from build123d import *

# Parameters (mm, degrees)
F0_W     = 152.4
F0_H     = 76.2
F1_DEPTH = 50.8
F3_DEPTH = 152.401
F5_DEPTH = 76.201
F6_W     = 76.2
F6_H     = 12.7
F7_DEPTH = 76.201


with BuildPart() as f1:
    # F0 (on Top) → F1 (new body)
    with BuildSketch(Plane.XY):
        Rectangle(F0_W, F0_H)
    extrude(amount=F1_DEPTH)

    # F2 (on face) → F3 (cut, through all)
    with BuildSketch(Plane.YZ.offset(76.2)):
        Polygon((25.40207, 12.7), (-25.4, 12.7), (-12.7, 0), (12.70207, 0), align=None)
    extrude(amount=-F3_DEPTH, mode=Mode.SUBTRACT)

    # F4 (on face) → F5 (cut, through all)
    with BuildSketch(Plane.XZ.offset(38.1)):
        Polygon((-25.4, 50.8), (-50.8, 50.8), (-50.8, 38.1), (-63.5, 38.1), (-63.5, 25.4), (-12.7, 25.4), (-12.7, 38.1), (-25.4, 38.1), align=None)
    extrude(amount=-F5_DEPTH, mode=Mode.SUBTRACT)

    # F6 (on face) → F7 (cut, through all)
    with BuildSketch(Plane.XZ.offset(38.1)):
        with Locations((38.1, 44.45)):
            Rectangle(F6_W, F6_H)
        Polygon((0, 38.1), (0, 50.8), (-7.272681, 50.8), align=None)
    extrude(amount=-F7_DEPTH, mode=Mode.SUBTRACT)


solid = f1.part
Can you work these out from the model? Positions are in its coordinate system, mm. A direction names the side the tool comes from. Give positions to 0.01 mm unless a question says otherwise; leave off trailing zeros. Order: outer loops, then holes, each group sorted by start corner. A loop starts at its lowest first (then second) coordinate and runs counter-clockwise, first axis right, second up. Notation, with made-up numbers: M 36.5,55 L 90.5,55 A13 ccw 90.5,73 Z; hole C -16,-5 d2. An arc over 180 degrees is marked long. Use one line per item in the form item = value. Start each with the question number.
Item 1: For faces 1 (the flat face through (-3.69, -0.53, 44.54)), 2 (the flat face through (-57, -1, 38.1)), 3 (the flat face through (-50.8, -1, 45)), 4 (the flat face through (1.1, 19, 6.3)), which set-ups out of +Z, -Z, +X, -X, +Y, -Y let a thin tool reach every point of the face, with its end or its side?
Item 2: If I drill on line 1 along X through (y, z) = (-8, 32.5); line 2 along Z through (x, y) = (-59.5, -4); line 3 along Z through (x, y) = (-18, 24.5), over which ranges is the centre line in solid material (lowest first)?
Item 3: If we section it at A-A (x = -52.5): Write out the boundary of the cut face in (y, z), then the cut area to 3 significant figures.
Item 4: If we section it at B-B (z = 8): Write out the boundary of the cut face in (x, y).
Item 5: If we section it at D-D (x = -10): Write out the boundary of the cut face in (y, z).
Item 6: If we section it at C-C (y = 18.5): Write out the boundary of the cut face in (x, z), then the cut area to 3 significant figures.
Item 7: We'd pull the mould along Y, two halves only. Please class faces 5 (the flat face through (-1, -38.1, 19)), 6 (the flat face through (1, 0, 12.7)), 7 (the flat face through (-1, -25, 0)): +Y half, -Y half, draft (parallel to the pull), parting line (faces both ways), or undercut.
Item 8: Will these pins go through, and if not, where does the flat tip stop? pin 1 Ø4 at (x, y) = (-20.5, -2) entering from -Z; pin 2 Ø3 at (x, y) = (-29, 11.5) entering from +Z; pin 3 Ø2 at (x, y) = (5, 26.5) entering from +Z.
Outcome:
q1.face_1 = +Z, +X, +Y, -Y
q1.face_2 = +Y, -Y
q1.face_3 = +Z, +Y, -Y
q1.face_4 = +X, -X
q2.line_1 = -76.2 to -63.5, -12.7 to 76.2
q2.line_2 = 12.7 to 25.4, 38.1 to 50.8
q2.line_3 = 0 to 11.8, 12.7 to 25.4, 38.1 to 50.8
q3.outline = M -38.1,0 L -12.7,0 L -25.4,12.7 L 25.4,12.7 L 12.7,0 L 38.1,0 L 38.1,25.4 L -38.1,25.4 Z; M -38.1,38.1 L 38.1,38.1 L 38.1,50.8 L -38.1,50.8 Z
q3.area = 2,420 mm2
q4.outline = M -76.2,-38.1 L 76.2,-38.1 L 76.2,-20.7 L -76.2,-20.7 Z; M -76.2,20.7 L 76.2,20.7 L 76.2,38.1 L -76.2,38.1 Z
q5.outline = M -38.1,0 L -12.7,0 L -25.4,12.7 L 25.4,12.7 L 12.7,0 L 38.1,0 L 38.1,50.8 L -38.1,50.8 Z
q6.outline = M -76.2,0 L 76.2,0 L 76.2,5.8 L -76.2,5.8 Z; M -76.2,12.7 L 76.2,12.7 L 76.2,38.1 L 0,38.1 L -7.27,50.8 L -25.4,50.8 L -25.4,38.1 L -12.7,38.1 L -12.7,25.4 L -63.5,25.4 L -63.5,38.1 L -50.8,38.1 L -50.8,50.8 L -76.2,50.8 Z
q6.area = 4,710 mm2
q7.face_5 = -Y half
q7.face_6 = undercut
q7.face_7 = draft
q8.pin_1 = 12.7
q8.pin_2 = 25.4
q8.pin_3 = 38.1
